Geometry check sheet. Reference: the model listing, model coordinates, mm. Face numbers are marked on the shaded views. Coordinates: 2 decimals unless noted, no trailing zeros. Order: outer loops, then holes, each group sorted by start corner. A loop starts at its lowest first (then second) coordinate and runs counter-clockwise, first axis right, second up. Notation, with made-up numbers: M -39.5,13.5 L -15.5,13.5 A19 cw -15.5,37.5 Z; hole C 62.5,65 d8. An arc over 180 degrees is marked long. One line per item, written item: value. Start each with the question number.
1) Sectioned sample at D-D, the plane x = -14. Enter the section's corners in (y, z), then the cut area to 3 significant figures.
2) Sectioned sample at A-A, the plane z = 0. Enter the section's corners in (x, y), then the cut area to 3 significant figures.
3) Sectioned sample at B-B, the plane x = 0. Enter the section's corners in (y, z), then the cut area to 3 significant figures.
4) Sectioned sample at C-C, the plane y = 5.5. Enter the section's corners in (x, z).
5) Go/stop test with flat-tipped pins: P1, Ø3, axis at y = 8, z = -34, coming from the -X side; P2, Ø1.5, axis at y = 2, z = -3.5, coming from the +X side; P3, Ø21, axis at x = 0, z = 0, coming from the -Y side; P4, Ø5, axis at y = 9, z = -3.5, coming from the +X side. Record where each tip stops, or that it passes through.
6) Draft check along X on the marked faces 1, 2, 3 and 4. Enter one of: pulls with the +X half, pulls with the -X half, needs draft (parallel to the pull), parting line crosses it, or undercut.
7) Thickness scan on L1, parallel to Z at x = -5, y = 2.5; L2, parallel to X at y = 4.5, z = 0; L3, parallel to X at y = 6.25, z = 39. Record the ranges inside material, lowest first. Write a range as from..to.
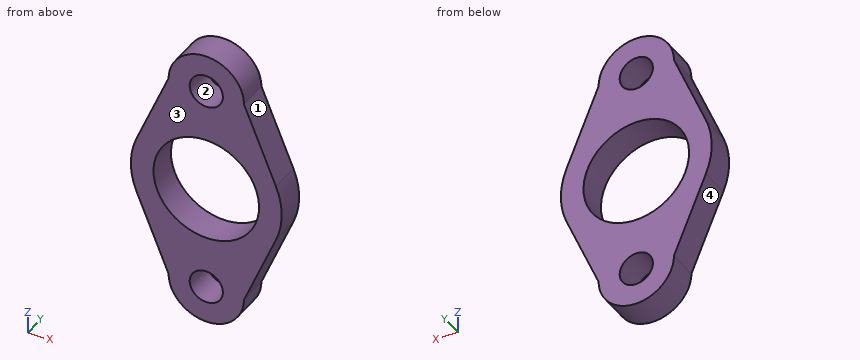
```python
from build123d import *

# Parameters (mm, degrees)
SKETCH2_R           = 20
SKETCH2_R_2         = 5.5
SKETCH2_R_3         = 17.5
BOSS_EXTRUDE3_DEPTH = 10


with BuildPart() as part:
    # Sketch2 → Boss-Extrude3 (new body)
    # profile 1 of 2: a face of its own
    with BuildSketch(Plane(origin=(0, 0, 0), x_dir=(1, 0, 0), z_dir=(0, 1, 0))):
        with BuildLine():
            Line((-12.5, 35), (-23.076923077, 9.615384615))
            ThreePointArc((-23.076923077, 9.615384615), (-25, 0), (-23.076923077, -9.615384615))
            Line((-23.076923077, -9.615384615), (-12.5, -35))
            ThreePointArc((-12.5, -35), (0, -47.5), (12.5, -35))
            Line((12.5, -35), (23.076923077, -9.615384615))
            ThreePointArc((23.076923077, -9.615384615), (25, 0), (23.076923077, 9.615384615))
            Line((23.076923077, 9.615384615), (12.5, 35))
            ThreePointArc((12.5, 35), (0, 47.5), (-12.5, 35))
        make_face()
        Circle(SKETCH2_R, mode=Mode.SUBTRACT)
        with Locations(Location((0, 35, 0), (0, 0, 270))):
            Circle(SKETCH2_R_2, mode=Mode.SUBTRACT)
        with Locations(Location((0, -35, 0), (0, 0, 270))):
            Circle(SKETCH2_R_2, mode=Mode.SUBTRACT)
    # profile 2 of 2: a face of its own
    with BuildSketch(Plane(origin=(0, 0, 0), x_dir=(1, 0, 0), z_dir=(0, 1, 0))):
        Circle(SKETCH2_R)
        with Locations(Location((0, 0, 0), (0, 0, 270))):
            Circle(SKETCH2_R_3, mode=Mode.SUBTRACT)
    extrude(amount=BOSS_EXTRUDE3_DEPTH)


solid = part.part
```
Final values:
1. outline: M 0,-31.4 L 10,-31.4 L 10,-10.5 L 0,-10.5 Z; M 0,10.5 L 10,10.5 L 10,31.4 L 0,31.4 Z
1. area: 418 mm^2
2. outline: M -25,0 L -17.5,0 L -17.5,10 L -25,10 Z; M 17.5,0 L 25,0 L 25,10 L 17.5,10 Z
2. area: 150 mm^2
3. outline: M 0,-47.5 L 10,-47.5 L 10,-40.5 L 0,-40.5 Z; M 0,-29.5 L 10,-29.5 L 10,-17.5 L 0,-17.5 Z; M 0,17.5 L 10,17.5 L 10,29.5 L 0,29.5 Z; M 0,40.5 L 10,40.5 L 10,47.5 L 0,47.5 Z
3. area: 380 mm^2
4. outline: M -23.08,-9.62 L -12.5,-35 A12.5 ccw 12.5,-35 L 23.08,-9.62 A25 ccw 23.08,9.62 L 12.5,35 A12.5 ccw -12.5,35 L -23.08,9.62 A25 ccw Z; hole C 0,0 d35; hole C 0,-35 d11; hole C 0,35 d11
5. P1: stops at x = -13.54
5. P2: stops at x = 24.85
5. P3: passes through
5. P4: stops at x = 24.98
6. face 1: pulls with the +X half
6. face 2: undercut
6. face 3: needs draft
6. face 4: pulls with the -X half
7. L1: z = -46.46..-37.29, -32.71..-16.77, 16.77..32.71, 37.29..46.46
7. L2: x = -25..-17.5, 17.5..25
7. L3: x = -11.84..-3.77, 3.77..11.84
